Autodesk Inventor part; units mm, degrees
ref_plane "YZ Plane" through (0, 0, 0) normal (1, 0, 0) x (0, 1, 0)
ref_plane "XZ Plane" through (0, 0, 0) normal (0, 1, 0) x (-1, 0, 0)
ref_plane "XY Plane" through (0, 0, 0) normal (0, 0, 1) x (1, 0, 0)
sketch "Sketch1" plane through (0, 0, 0) normal (1, 0, 0) x (0, 1, 0)
  line L0 (0, 0) -> (83.185, 0)
  line L1 (83.185, 0) -> (83.185, -50.8)
  line L2 (83.185, -50.8) -> (0, -50.8)
  line L3 (0, -50.8) -> (0, 0)
  arc A0 (57.785, -44.45) -> (57.785, -6.35) centre (57.785, -25.4) ccw
  arc A1 (14.2875, -6.35) -> (6.35, -14.2875) centre (14.2875, -14.2875) ccw
  arc A2 (6.35, -36.5125) -> (14.2875, -44.45) centre (14.2875, -36.5125) ccw
  line L4 (14.2875, -44.45) -> (57.785, -44.45)
  line L5 (14.2875, -6.35) -> (57.785, -6.35)
  line L6 (6.35, -14.2875) -> (6.35, -36.5125)
  line L7 (57.785, 0) -> (57.785, -50.8)
  circle A3 centre (37.465, -3.175) radius 1.7145
  circle A4 centre (37.465, -47.625) radius 1.7145
  circle A5 centre (5.08, -45.72) radius 1.7145
  circle A6 centre (5.08, -5.08) radius 1.7145
  circle A7 centre (78.105, -5.08) radius 1.7145
  circle A8 centre (78.105, -45.72) radius 1.7145
  dimension "d0" = 83.185
  dimension "d1" = 50.8
  dimension "d2" = 38.1
  dimension "d3" = 25.4
  dimension "d4" = 25.4
  dimension "d5" = 15.875
  dimension "d6" = 15.875
  dimension "d7" = 14.2875
  dimension "d8" = 14.2875
  dimension "d9" = 14.2875
  dimension "d10" = 14.2875
  dimension "d19" = 25.4
  dimension "d20" = 3.175
  dimension "d21" = 3.175
  dimension "d28" = 3.429
  dimension "d29" = 5.08
  dimension "d30" = 5.08
  dimension "d31" = 45.72
  dimension "d32" = 45.72
  dimension "d33" = 3.429
  dimension "d34" = 3.429
  dimension "d35" = 5.08
  dimension "d36" = 5.08
  dimension "d37" = 5.08
  dimension "d38" = 5.08
  dimension "d39" = 5.08
  dimension "d40" = 5.08
extrude "Extrusion1" add sketch "Sketch1" against normal blind 3.175 contours L0 L7 L5 A1 L6 A2 L4 L2 L3 | L0 L1 L2 L7 A0
properties part number "Engine Head Gasket"
Could you check a few things on this model? Use its own coordinates, in mm. A direction names the side the tool comes from. Round coordinates to 2 decimals unless told otherwise and drop trailing zeros. Order: outer loops, then holes, each group sorted by start corner. A loop starts at its lowest first (then second) coordinate and runs counter-clockwise, first axis right, second up. Notation, with made-up numbers: M -19,75 L 36,75 A32 ccw 36,114 Z; hole C 44.25,-8.75 d1. An arc over 180 degrees is marked long. One line per item, written item: value.
(1) Imagine slicing it at C-C (y = 34). Write out the boundary of the cut face in (x, z) (3 decimals), and give its area (3 significant figures).
Ans:
outline: M -3.175,-50.8 L 0,-50.8 L 0,-44.45 L -3.175,-44.45 Z; M -3.175,-6.35 L 0,-6.35 L 0,0 L -3.175,0 Z
area: 40.3 mm^2
(2) I need wall thicknesses on line 1 along Z through (x, y) = (-1.55, 5.08); line 2 along Z through (x, y) = (-3, 52.5); line 3 along Z through (x, y) = (-0.35, 37). Which ranges of each line are inside material? Lowest first, please. Write a range as from..to.
Ans:
line 1: z = -50.8..-47.43, -44.01..-6.79, -3.37..0
line 2: z = -50.8..-44.45, -6.35..0
line 3: z = -50.8..-49.28, -45.97..-44.45, -6.35..-4.83, -1.52..0
(3) If we mould it in two halves opening along Z, with no side actions, what happens to faces 1 (the cylindrical face through (-1.57, 8.61, -42.06)), 2 (the flat face through (0, 41, -48)), 3 (the flat face through (-2, 41, 0))? For each: released by +Z, released by -Z, zero draft, split by the parting line, or undercut.
Ans:
face 1: undercut
face 2: zero draft
face 3: released by +Z
(4) Imagine slicing it at D-D (x = -1.6). Count the separate pieces of the cut face and the enclosed holes in it, and give its area (3 significant figures).
Ans:
separate pieces: 1
enclosed holes: 7
area: 1,670 mm^2
(5) Imagine slicing it at A-A (y = 5.08). Write out the boundary of the cut face in (x, z) (1 decimal).
Ans:
outline: M -3.2,-50.8 L 0,-50.8 L 0,-47.4 L -3.2,-47.4 Z; M -3.2,-44 L 0,-44 L 0,-6.8 L -3.2,-6.8 Z; M -3.2,-3.4 L 0,-3.4 L 0,0 L -3.2,0 Z
(6) I'm going to push a flat-ended pin straight in: P1, Ø2.5, axis at y = 78.105, z = -45.72, coming from the +X side. Where does the tip first touch, or does it pass through?
Ans:
P1: passes through
(7) Imagine slicing it at B-B (z = -25.4). Write out the boundary of the cut face in (x, y) (3 decimals).
Ans:
outline: M -3.175,0 L 0,0 L 0,6.35 L -3.175,6.35 Z; M -3.175,76.835 L 0,76.835 L 0,83.185 L -3.175,83.185 Z
(8) Which directions (+Z, -Z, +X, -X, +Y, -Y) give clear straight access to the entire face, cutting with the end or side of a thin tool? Please do faces 4 (the cylindrical face through (-1.57, 76.83, -25.82)), 5 (the flat face through (-2, 0, -26)).
Ans:
face 4: +X, -X
face 5: +Z, -Z, +X, -X, -Y
